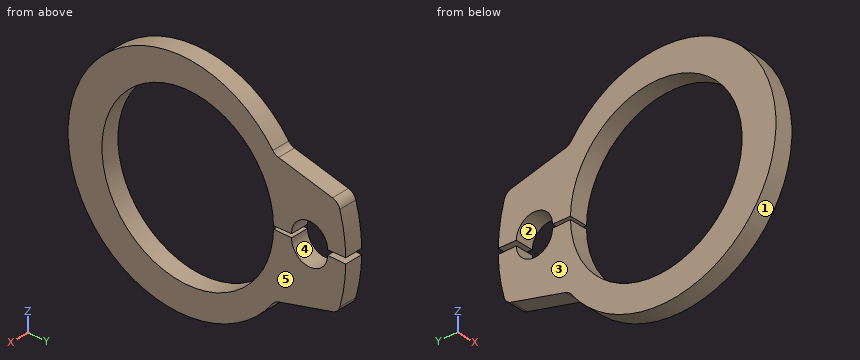
```python
from build123d import *

# Parameters (mm, degrees)
EXTRUDE1_DEPTH = 0.4
FILLET1_R      = 0.45


with BuildPart() as part:
    # Sketch1 → Extrude1 (new body, symmetric)
    with BuildSketch(Plane(origin=(0, 0, 0), x_dir=(0, 0, -1), z_dir=(1, 0, 0))):
        with BuildLine():
            Line((0.066319144, 3.799421242), (0.08028107, 4.599299398))
            ThreePointArc((0.08028107, 4.599299398), (0.894121151, 5.385215629), (0.10820492, 6.19905571))
            Line((0.10820492, 6.19905571), (0.122166845, 6.998933866))
            ThreePointArc((0.122166845, 6.998933866), (1.151239086, 6.904683089), (2.155222001, 6.659956316))
            Line((2.155222001, 6.659956316), (2.853372649, 3.859827007))
            ThreePointArc((2.853372649, 3.859827007), (0, -5.3), (-2.853372649, 3.859827007))
            Line((-2.853372649, 3.859827007), (-2.155222001, 6.659956316))
            ThreePointArc((-2.155222001, 6.659956316), (-1.151239086, 6.904683089), (-0.122166845, 6.998933866))
            Line((-0.122166845, 6.998933866), (-0.10820492, 6.19905571))
            ThreePointArc((-0.10820492, 6.19905571), (-0.894121151, 5.385215629), (-0.08028107, 4.599299398))
            Line((-0.08028107, 4.599299398), (-0.066319144, 3.799421242))
            ThreePointArc((-0.066319144, 3.799421242), (0, -3.8), (0.066319144, 3.799421242))
        make_face()
    extrude(amount=EXTRUDE1_DEPTH, both=True)

    # Fillet1
    fillet1_edges = [part.edges().sort_by_distance(p)[0] for p in [
        (0, 6.659956316, -2.155222001),
        (0, 3.859827007, -2.853372649),
        (0, 3.859827007, 2.853372649),
        (0, 6.659956316, 2.155222001),
    ]]
    fillet(fillet1_edges, radius=FILLET1_R)


solid = part.part
```
Can you work these out from the model? Positions are in its coordinate system, mm. Face numbers are marked on the shaded views. A direction names the side the tool comes from. Round coordinates to 2 decimals unless told otherwise and drop trailing zeros. Loops run counter-clockwise (first coordinate to the right, second up) from the corner with the lowest first, then second, coordinate; pieces in that order, holes last.
Item 1: If we mould it in two halves opening along Z, with no side actions, what happens to the marked faces 1, 2 and 3? For each: +Z half, -Z half, draft (parallel to the pull), parting line (faces both ways), or undercut.
Item 2: Suppose I cut it at C-C, the plane x = -0.2. Write out the boundary of the cut face in (y, z), then the cut area to 3 significant figures.
Item 3: Suppose I cut it at D-D, the plane z = -0.25. Write out the boundary of the cut face in (x, y).
Item 4: Which directions (+Z, -Z, +X, -X, +Y, -Y) give clear straight access to the entire face, cutting with the end or side of a thin tool? Please do the marked faces 4 and 5.
Item 5: Please list where these lines run through material, in increasing order: L1, parallel to Y at x = -0.1, z = -0.25; L2, parallel to Z at x = 0.25, y = 0; L3, parallel to Z at x = 0, y = 1.25.
Item 6: Suppose I cut it at B-B, the plane z = -1.5. Write out the boundary of the cut face in (x, y), then the cut area to 3 significant figures.
Item 7: Suppose I cut it at A-A, the plane y = 2.25. Write out the boundary of the cut face in (x, z).
Reported:
1. face 1: parting line
1. face 2: undercut
1. face 3: draft
2. outline: (3.77, -2.98) arc R0.45 cw to (4.02, -2.81) - (6.41, -2.22) arc R0.45 ccw to (6.74, -1.9) arc R7 ccw to (7, -0.12) - (6.2, -0.11) arc R0.8 cw to (4.6, -0.08) - (3.8, -0.07) arc R3.8 cw (long way) to (3.8, 0.07) - (4.6, 0.08) arc R0.8 cw to (6.2, 0.11) - (7, 0.12) arc R7 ccw to (6.74, 1.9) arc R0.45 ccw to (6.41, 2.22) - (4.02, 2.81) arc R0.45 cw to (3.77, 2.98) arc R5.02 ccw (long way) to start
2. area: 42.9 mm2
3. outline: (-0.4, -5.29) - (0.4, -5.29) - (0.4, -3.79) - (-0.4, -3.79) - close; (-0.4, 3.79) - (0.4, 3.79) - (0.4, 4.61) - (-0.4, 4.61) - close; (-0.4, 6.18) - (0.4, 6.18) - (0.4, 7) - (-0.4, 7) - close
4. face 4: +X, -X
4. face 5: +Z, -Z, +X, +Y, -Y
5. L1: y = -5.29 to -3.79, 3.79 to 4.61, 6.18 to 7
5. L2: z = -5.02 to -3.8, 3.8 to 5.02
5. L3: z = -4.79 to -3.59, 3.59 to 4.79
6. outline: (-0.4, -5.07) - (0.4, -5.07) - (0.4, -3.49) - (-0.4, -3.49) - close; (-0.4, 3.49) - (0.4, 3.49) - (0.4, 6.84) - (-0.4, 6.84) - close
6. area: 3.94 mm2
7. outline: (-0.4, -4.34) - (0.4, -4.34) - (0.4, -3.06) - (-0.4, -3.06) - close; (-0.4, 3.06) - (0.4, 3.06) - (0.4, 4.34) - (-0.4, 4.34) - close
